Read the model definition and answer for the solid it produces. Units are mm, in the model's axes. Face numbers are marked on the shaded views. A direction names the side the tool comes from. Coordinates: 2 decimals unless noted, no trailing zeros. Write each loop counter-clockwise with the first axis right and the second up, starting at its lowest first coordinate (ties: lowest second). Pieces come first, ordered by that corner, then holes.
1) This flat-tipped pin is pushed along its axis until it touches: pin 1 Ø0.6 at (x, z) = (0, 1.5) entering from +Y. Where does it stop, or does it pass through?
2) Find the intervals of material crossed by line 1 (X direction, y = 9.25, z = 0.9) (3 decimals); line 2 (Y direction, x = 2.5, z = 1.45); line 3 (Y direction, x = -6.5, z = 0.2), in increasing order.
3) The part is cut by section B-B (y = -6). Determine the outline of the cut face in (x, z).
4) Which of the six approach directions +Z, -Z, +X, -X, +Y, -Y give full straight-line access (tool end or side, diameter ignored) to the marked faces 4, 5, 6, 7 and 8?
5) The part is cut by section A-A (x = -1.25). Determine the outline of the cut face in (y, z).
6) Determine the mould class of the marked faces 1, 2 and 3 for opening direction X: +X half, -X half, draft (parallel to the pull), parting line (faces both ways), or undercut.
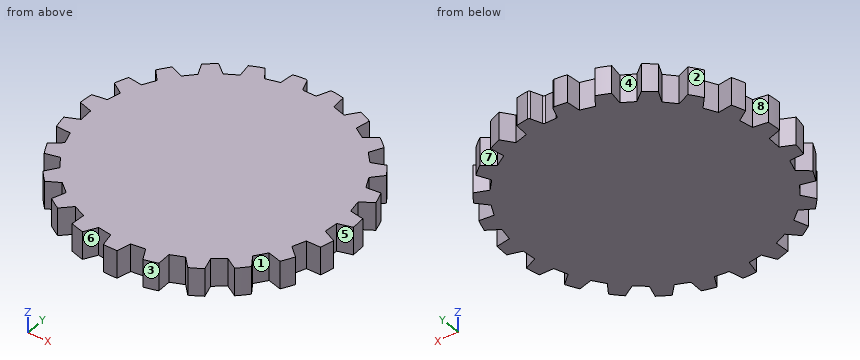
from build123d import *

# Parameters (mm, degrees)
F0_R     = 10
F1_DEPTH = 2
F3_DEPTH = 25
F4_COUNT = 23
F5_R     = 0.15


with BuildPart() as f1:
    # F0 (on Top) → F1 (new body)
    with BuildSketch(Plane.XY):
        Circle(F0_R)
    extrude(amount=F1_DEPTH)

    # F2 (on face) → F3 (cut)
    with BuildSketch(Plane.XY.offset(2)):
        with BuildLine():
            Line((0, 10), (0, 9))
            Line((0, 9), (0.5, 9))
            Line((0.5, 9), (0.8657328431, 9.9624548503))
            ThreePointArc((0.8657328431, 9.9624548503), (0.4332732954, 9.9906093033), (0, 10))
        make_face()
        with BuildLine():
            Line((-0.5, 9), (0, 9))
            Line((0, 9), (0, 10))
            ThreePointArc((0, 10), (-0.4332732954, 9.9906093033), (-0.8657328431, 9.9624548503))
            Line((-0.8657328431, 9.9624548503), (-0.5, 9))
        make_face()
    f3 = extrude(amount=-F3_DEPTH, mode=Mode.SUBTRACT)

    # F4: F3 ×23 about axis
    f4_axis = Axis((0, 0, 0), (0, 0, -1))
    for i in range(1, F4_COUNT):
        add(f3.rotate(f4_axis, i * 360 / F4_COUNT), mode=Mode.SUBTRACT)

    # F5
    f5_edges = [f1.edges().sort_by_distance(p)[0] for p in [
        (0.5, 9, 1),
        (-0.5, 9, 1),
        (0.865733, 9.962455, 1),
        (-0.865733, 9.962455, 1),
    ]]
    fillet(f5_edges, radius=F5_R)


solid = f1.part
Reported:
1. pin 1: stops at y = 9
2. line 1: x = -3.8 to -3.441, -1.906 to -0.595, 0.595 to 1.906, 3.441 to 3.8
2. line 2: y = -9.68 to 8.65
2. line 3: y = -6.92 to 6.23, 7.05 to 7.6
3. outline: (-7.33, 0) - (7.33, 0) - (7.33, 2) - (-7.33, 2) - close
4. face 4: +Z, -Z
4. face 5: +Z, -Z, +X
4. face 6: +Z, -Z, -Y
4. face 7: +Z, -Z, +Y
4. face 8: +Z, -Z, -X
5. outline: (-8.91, 0) - (9.92, 0) - (9.92, 2) - (-8.91, 2) - close
6. face 1: undercut
6. face 2: -X half
6. face 3: +X half
